For this review, take the finished solid that the model builds, in its own axes (mm). Round coordinates to 2 decimals unless told otherwise and drop trailing zeros. Order: outer loops, then holes, each group sorted by start corner. A loop starts at its lowest first (then second) coordinate and runs counter-clockwise, first axis right, second up. Notation, with made-up numbers: (15, 71) - (27, 71) arc R3 cw to (27, 76) - close; hole circle Ø2 at (-6, 4.5). An arc over 180 degrees is marked (long way). One line per question, with ' | ' between items.
```python
from build123d import *

# Parameters (mm, degrees)
SKETCH1_W           = 400
SKETCH1_H           = 400
BOSS_EXTRUDE1_DEPTH = 7.5
CHAMFER1_SIZE       = 10
SKETCH3_R           = 8
CUT_EXTRUDE1_DEPTH  = 16


with BuildPart() as part:
    # Sketch1 → Boss-Extrude1 (new body, symmetric)
    with BuildSketch(Plane(origin=(0, 0, 0), x_dir=(1, 0, 0), z_dir=(0, 1, 0))):
        with Locations((200, 200)):
            Rectangle(SKETCH1_W, SKETCH1_H)
    extrude(amount=BOSS_EXTRUDE1_DEPTH, both=True)

    # Chamfer1
    chamfer1_edges = [part.edges().sort_by_distance(p)[0] for p in [
        (0, 0, -400),
        (400, 0, -400),
        (400, 0, 0),
        (0, 0, 0),
    ]]
    chamfer(chamfer1_edges, length=CHAMFER1_SIZE)

    # Sketch3 → Cut-Extrude1 (cut)
    with BuildSketch(Plane(origin=(0, 7.5, 0), x_dir=(1, 0, 0), z_dir=(0, 1, 0))):
        with Locations((307.5, 307.5)):
            Circle(SKETCH3_R)
        with Locations((307.5, 92.5)):
            Circle(SKETCH3_R)
        with Locations((92.5, 92.5)):
            Circle(SKETCH3_R)
        with Locations((92.5, 307.5)):
            Circle(SKETCH3_R)
    extrude(amount=-CUT_EXTRUDE1_DEPTH, mode=Mode.SUBTRACT)


solid = part.part
```
(1) For probe 1 along Z at (x, y) = (307.5, 2); probe 2 along X at (y, z) = (-0.75, -92.5); probe 3 along Z at (x, y) = (305, 3.75), list the stretches that pass through material, from the lowest coordinate up. Write a range as [from, to].
Output values:
probe 1: [-400, -315.5], [-299.5, -100.5], [-84.5, 0] | probe 2: [0, 84.5], [100.5, 299.5], [315.5, 400] | probe 3: [-400, -315.1], [-299.9, -100.1], [-84.9, 0]
(2) We need section A-A on z = -307.5. State the section outline as (x, y) points.
Output values:
outline: (0, -7.5) - (84.5, -7.5) - (84.5, 7.5) - (0, 7.5) - close; (100.5, -7.5) - (299.5, -7.5) - (299.5, 7.5) - (100.5, 7.5) - close; (315.5, -7.5) - (400, -7.5) - (400, 7.5) - (315.5, 7.5) - close
(3) We need section B-B on x = 307.5. State the section outline as (y, z) points, plus the area to 3 significant figures.
Output values:
outline: (-7.5, -400) - (7.5, -400) - (7.5, -315.5) - (-7.5, -315.5) - close; (-7.5, -299.5) - (7.5, -299.5) - (7.5, -100.5) - (-7.5, -100.5) - close; (-7.5, -84.5) - (7.5, -84.5) - (7.5, 0) - (-7.5, 0) - close | area: 5,520 mm^2
(4) Insertion check: pin 1 (13 mm diameter, centred on x = 307.5, z = -92.5, fed in from +Y). The pin has a flat end and moves straight along its axis. Give the tip position at first contact, or say it passes through.
Output values:
pin 1: through
(5) Mouldability with a two-part tool opening along X and no side actions: class faces 1 (the flat face through (5, 0, -5)), 2 (the flat face through (197, -7.5, -203)), 3 (the flat face through (395, 0, -395)), 4 (the cylindrical face through (86.151, 0.105, -87.632)) as released by +X, released by -X, zero draft, split by the parting line, or undercut.
Output values:
face 1: released by -X | face 2: zero draft | face 3: released by +X | face 4: undercut
